Can you work these out from the model? Positions are in its coordinate system, mm. Face numbers are marked on the shaded views. Round coordinates to 2 decimals unless told otherwise and drop trailing zeros. Order: outer loops, then holes, each group sorted by start corner. A loop starts at its lowest first (then second) coordinate and runs counter-clockwise, first axis right, second up.
from build123d import *

# Parameters (mm, degrees)
SKETCH1_W           = 73
SKETCH1_H           = 60
BOSS_EXTRUDE1_DEPTH = 16.9
FILLET1_R           = 15
CUT_EXTRUDE1_REACH  = 57.087
SKETCH2_R           = 21
SKETCH3_W           = 40
SKETCH3_H           = 20
CUT_EXTRUDE2_DEPTH  = 6.2
CUT_EXTRUDE3_REACH  = 57.087
SKETCH4_R           = 1
SKETCH5_R           = 2.5
CUT_EXTRUDE4_DEPTH  = 2


with BuildPart() as part:
    # Sketch1 → Boss-Extrude1 (new body)
    with BuildSketch(Plane(origin=(0, 0, 0), x_dir=(1, 0, 0), z_dir=(0, 1, 0))):
        with Locations((6.5, 0)):
            Rectangle(SKETCH1_W, SKETCH1_H)
    extrude(amount=BOSS_EXTRUDE1_DEPTH)

    # Fillet1
    fillet1_edges = [part.edges().sort_by_distance(p)[0] for p in [
        (-30, 8.45, -30),
        (-30, 8.45, 30),
    ]]
    fillet(fillet1_edges, radius=FILLET1_R)

    # Sketch2 → Cut-Extrude1 (cut, up to next)
    with BuildSketch(Plane(origin=(0, 16.9, 0), x_dir=(1, 0, 0), z_dir=(0, 1, 0)), mode=Mode.PRIVATE) as cut_extrude1_sk1:
        with Locations(Location((10.5, -0.1, 0), (0, 0, 270))):
            Circle(SKETCH2_R)
    cut_extrude1_tool1 = extrude(cut_extrude1_sk1.sketch, amount=-CUT_EXTRUDE1_REACH, mode=Mode.PRIVATE) & part.part
    add(cut_extrude1_tool1.solids().sort_by_distance((10.5, 16.9, 0.1))[0], mode=Mode.SUBTRACT)

    # Sketch3 → Cut-Extrude2 (cut)
    with BuildSketch(Plane.XZ):
        with Locations((-10, 0)):
            Rectangle(SKETCH3_W, SKETCH3_H)
    extrude(amount=-CUT_EXTRUDE2_DEPTH, mode=Mode.SUBTRACT)

    # Sketch4 → Cut-Extrude3 (cut, up to next)
    with BuildSketch(Plane(origin=(0, 16.9, 0), x_dir=(1, 0, 0), z_dir=(0, 1, 0)), mode=Mode.PRIVATE) as cut_extrude3_sk1:
        with Locations(Location((34, 20, 0), (0, 0, 270))):
            Circle(SKETCH4_R)
    cut_extrude3_tool1 = extrude(cut_extrude3_sk1.sketch, amount=-CUT_EXTRUDE3_REACH, mode=Mode.PRIVATE) & part.part
    # Sketch4 → Cut-Extrude3 (cut, up to next)
    with BuildSketch(Plane(origin=(0, 16.9, 0), x_dir=(1, 0, 0), z_dir=(0, 1, 0)), mode=Mode.PRIVATE) as cut_extrude3_sk2:
        with Locations(Location((34, -20, 0), (0, 0, 270))):
            Circle(SKETCH4_R)
    cut_extrude3_tool2 = extrude(cut_extrude3_sk2.sketch, amount=-CUT_EXTRUDE3_REACH, mode=Mode.PRIVATE) & part.part
    # Sketch4 → Cut-Extrude3 (cut, up to next)
    with BuildSketch(Plane(origin=(0, 16.9, 0), x_dir=(1, 0, 0), z_dir=(0, 1, 0)), mode=Mode.PRIVATE) as cut_extrude3_sk3:
        with Locations(Location((-19, -20, 0), (0, 0, 270))):
            Circle(SKETCH4_R)
    cut_extrude3_tool3 = extrude(cut_extrude3_sk3.sketch, amount=-CUT_EXTRUDE3_REACH, mode=Mode.PRIVATE) & part.part
    # Sketch4 → Cut-Extrude3 (cut, up to next)
    with BuildSketch(Plane(origin=(0, 16.9, 0), x_dir=(1, 0, 0), z_dir=(0, 1, 0)), mode=Mode.PRIVATE) as cut_extrude3_sk4:
        with Locations(Location((-19, 20, 0), (0, 0, 270))):
            Circle(SKETCH4_R)
    cut_extrude3_tool4 = extrude(cut_extrude3_sk4.sketch, amount=-CUT_EXTRUDE3_REACH, mode=Mode.PRIVATE) & part.part
    add(cut_extrude3_tool1.solids().sort_by_distance((34, 16.9, -20))[0], mode=Mode.SUBTRACT)
    add(cut_extrude3_tool2.solids().sort_by_distance((34, 16.9, 20))[0], mode=Mode.SUBTRACT)
    add(cut_extrude3_tool3.solids().sort_by_distance((-19, 16.9, 20))[0], mode=Mode.SUBTRACT)
    add(cut_extrude3_tool4.solids().sort_by_distance((-19, 16.9, -20))[0], mode=Mode.SUBTRACT)

    # Sketch5 → Cut-Extrude4 (cut)
    with BuildSketch(Plane(origin=(0, 16.9, 0), x_dir=(1, 0, 0), z_dir=(0, 1, 0))):
        with Locations(Location((-19, 20, 0), (0, 0, 270))):
            Circle(SKETCH5_R)
        with Locations(Location((-19, -20, 0), (0, 0, 270))):
            Circle(SKETCH5_R)
        with Locations(Location((34, -20, 0), (0, 0, 270))):
            Circle(SKETCH5_R)
        with Locations(Location((34, 20, 0), (0, 0, 270))):
            Circle(SKETCH5_R)
    extrude(amount=-CUT_EXTRUDE4_DEPTH, mode=Mode.SUBTRACT)


solid = part.part
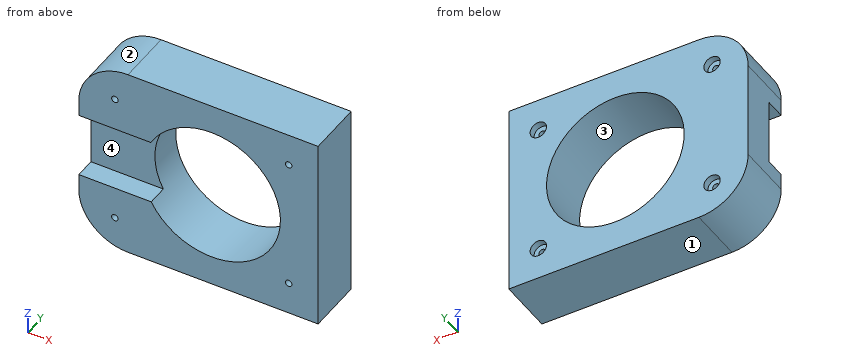
(1) I want a section at B-B, the plane y = 1.5. List the corners of the cut face in (x, z) for me.
(2) I want a section at A-A, the plane x = 34. List the corners of the cut face in (y, z) for me, plus the area to 3 significant figures.
(3) Please list where these lines run through material, in increasing order: probe 1 along Z at (x, y) = (17.5, 13); probe 2 along Z at (x, y) = (28, 4.75); probe 3 along X at (y, z) = (3.25, -17.5).
(4) I want a section at D-D, the plane z = 0.1. List the corners of the cut face in (x, y) for me, plus the area to 3 significant figures.
(5) If we mould it in two halves opening along Z, with no side actions, what happens to the marked faces 1, 2, 3 and 4? For each: pulls with the +Z half, pulls with the -Z half, needs draft (parallel to the pull), parting line crosses it, or undercut.
(6) I want a section at C-C, the plane x = 10.5. List the corners of the cut face in (y, z) for me, plus the area to 3 significant figures.
(7) I'm going to push flat-ended pins straight in: pin 1 Ø4.5 at (x, z) = (-19, -20) entering from +Y; pin 2 Ø5 at (y, z) = (11.5, -19) entering from -X; pin 3 Ø4.5 at (x, z) = (34, 20) entering from -Y; pin 4 Ø5 at (x, y) = (-21, 3.5) entering from +Z. Where does each tip first touch, or does it pass through?
Ans:
1. outline: (-30, -15) arc R15 ccw to (-15, -30) - (43, -30) - (43, 30) - (-15, 30) arc R15 ccw to (-30, 15) - (-30, 10) - (-8.02, 10) arc R21 cw (long way) to (-7.91, -10) - (-30, -10) - close; hole circle Ø2 at (-19, -20); hole circle Ø2 at (-19, 20); hole circle Ø2 at (34, -20); hole circle Ø2 at (34, 20)
2. outline: (0, -30) - (16.9, -30) - (16.9, -22.5) - (14.9, -22.5) - (14.9, -21) - (0, -21) - close; (0, -19) - (14.9, -19) - (14.9, -17.5) - (16.9, -17.5) - (16.9, 17.5) - (14.9, 17.5) - (14.9, 19) - (0, 19) - close; (0, 21) - (14.9, 21) - (14.9, 22.5) - (16.9, 22.5) - (16.9, 30) - (0, 30) - close
2. area: 934 mm2
3. probe 1: z = -30 to -19.7, 19.9 to 30
3. probe 2: z = -30 to -11.51, 11.71 to 30
3. probe 3: x = -29.79 to -0.96, 21.96 to 43
4. outline: (-30, 6.2) - (-10.5, 6.2) - (-10.5, 16.9) - (-30, 16.9) - close; (31.5, 0) - (43, 0) - (43, 16.9) - (31.5, 16.9) - close
4. area: 403 mm2
5. face 1: pulls with the -Z half
5. face 2: pulls with the +Z half
5. face 3: undercut
5. face 4: undercut
6. outline: (0, -30) - (16.9, -30) - (16.9, -20.9) - (0, -20.9) - close; (0, 21.1) - (16.9, 21.1) - (16.9, 30) - (0, 30) - close
6. area: 304 mm2
7. pin 1: stops at y = 14.9
7. pin 2: stops at x = -29.92
7. pin 3: stops at y = 0
7. pin 4: stops at z = 29.59
